```python
from build123d import *

# Parameters (mm, degrees)
SKETCH_1_R          = 5
EXTRUDE_1_DEPTH     = 15.4
SKETCH_2_R          = 2.1
CUT_EXTRUDE_1_DEPTH = 10


with BuildPart() as part:
    # ｽｹｯﾁ1 → ﾎﾞｽ - 押し出し1 (new body)
    with BuildSketch(Plane.XY):
        with Locations(Location((0, 0, 0), (0, 0, 180))):
            Circle(SKETCH_1_R)
    extrude(amount=EXTRUDE_1_DEPTH)

    # ｽｹｯﾁ2 → ｶｯﾄ - 押し出し1 (cut)
    with BuildSketch(Plane.XY.offset(15.4)):
        Circle(SKETCH_2_R)
    cut_extrude_1 = extrude(amount=-CUT_EXTRUDE_1_DEPTH, mode=Mode.SUBTRACT)

    # ﾐﾗｰ1: ｶｯﾄ - 押し出し1 across plane
    add(cut_extrude_1.mirror(Plane.XY.offset(7.7)), mode=Mode.SUBTRACT)


solid = part.part
```
Can you work these out from the model? Positions are in its coordinate system, mm. Round coordinates to 2 decimals unless told otherwise and drop trailing zeros. Loops run counter-clockwise (first coordinate to the right, second up) from the corner with the lowest first, then second, coordinate; pieces in that order, holes last.
Item 1: Suppose I cut it at D-D, the plane x = -4. Write out the boundary of the cut face in (y, z).
Item 2: Please list where these lines run through material, in increasing order: L1, parallel to Y at x = 0, z = 7.5; L2, parallel to X at y = 1.5, z = 9.5; L3, parallel to Y at x = -1.75, z = 10.
Item 3: Suppose I cut it at A-A, the plane y = 0. Write out the boundary of the cut face in (x, z), then the cut area to 3 significant figures.
Item 4: Will these pins go through, and if not, where does the flat tip stop? pin 1 Ø4 at (x, z) = (3.5, 10.5) entering from +Y; pin 2 Ø5 at (y, z) = (-3.5, 2) entering from -X; pin 3 Ø4 at (x, y) = (0, 0) entering from +Z.
Item 5: Suppose I cut it at C-C, the plane z = 4. Write out the boundary of the cut face in (x, y), then the cut area to 3 significant figures.
Item 6: If we mould it in two halves opening along X, with no side actions, what happens to faces 1 (the cylindrical face through (5, 0, 8)), 2 (the flat face through (-1, 2.2, 0)), 3 (the cylindrical face through (2.003, 0.631, 7.592))? For each: +X half, -X half, draft (parallel to the pull), parting line (faces both ways), or undercut.
Item 7: Suppose I cut it at B-B, the plane x = -1.5. Write out the boundary of the cut face in (y, z), then the cut area to 3 significant figures.
Reported:
1. outline: (-3, 0) - (3, 0) - (3, 15.4) - (-3, 15.4) - close
2. L1: y = -5 to -2.1, 2.1 to 5
2. L2: x = -4.77 to -1.47, 1.47 to 4.77
2. L3: y = -4.68 to -1.16, 1.16 to 4.68
3. outline: (-5, 0) - (-2.1, 0) - (-2.1, 15.4) - (-5, 15.4) - close; (2.1, 0) - (5, 0) - (5, 15.4) - (2.1, 15.4) - close
3. area: 89.3 mm2
4. pin 1: stops at y = 4.77
4. pin 2: stops at x = -4.9
4. pin 3: passes through
5. outline: circle Ø10 at (0, 0); hole circle Ø4.2 at (0, 0)
5. area: 64.7 mm2
6. face 1: parting line
6. face 2: draft
6. face 3: undercut
7. outline: (-4.77, 0) - (-1.47, 0) - (-1.47, 15.4) - (-4.77, 15.4) - close; (1.47, 0) - (4.77, 0) - (4.77, 15.4) - (1.47, 15.4) - close
7. area: 102 mm2
